Build history of the part. All positions in model axes, mm. Face numbers are marked on the shaded views. A direction names the side the tool comes from. Give positions to 0.01 mm unless a question says otherwise; leave off trailing zeros. Loops run counter-clockwise (first coordinate to the right, second up) from the corner with the lowest first, then second, coordinate; pieces in that order, holes last. Notation, with made-up numbers: (11.5, 9) -> (34.5, 9) arc R32 ccw to (34.5, 40) -> close; hole circle Ø11 at (58, -19.5). An arc over 180 degrees is marked (long way). One line per question, with ' | ' between items. Start each with the question number.
(1) Slice it at D-D, the plane z = 8. Write the cut outline in (x, y), then the cut area to 3 significant figures.
(2) Mould opens along X. For the marked faces 1, 2 and 3 say: pulls with the +X half, pulls with the -X half, needs draft (parallel to the pull), parting line crosses it, or undercut.
(3) Slice it at B-B, the plane z = 18. Write the cut outline in (x, y).
(4) 3-axis set-ups, long thin cutter, end or side, ignore diameter. For the marked faces 4 and 5: which of +Z, -Z, +X, -X, +Y, -Y reach the whole face in a straight line?
(5) Slice it at C-C, the plane x = 30. Write the cut outline in (y, z).
(6) Flat gauge pins, fed straight in: pin 1 Ø10 at (x, z) = (32.5, 14.5) entering from +Y; pin 2 Ø1.6 at (x, y) = (30, 1) entering from -Z; pin 3 Ø4 at (x, y) = (26.5, 20.5) entering from -Z; pin 4 Ø1 at (x, y) = (14.5, 12.5) entering from +Z. Where does each tip first touch, or does it go through?
(7) Slice it at A-A, the plane y = 23. Write the cut outline in (x, z).
(8) Drill centre lines: L1, parallel to X at y = 15, z = 16; L2, parallel to Z at x = 59.15, y = 56; L3, parallel to Z at x = 26.5, y = 25. Where is each one in solid material? Low to high. Write a range as from..to.
```python
from build123d import *

# Parameters (mm, degrees)
F0_W     = 60
F0_H     = 60
F1_DEPTH = 2
F3_DEPTH = 20
F5_DEPTH = 10
F6_R     = 2
F7_DEPTH = 69.4


with BuildPart() as f1:
    # F0 (on Top) → F1 (new body)
    with BuildSketch(Plane.XY):
        with Locations((30, 30)):
            Rectangle(F0_W, F0_H)
    extrude(amount=F1_DEPTH)

    # F2 (on face) → F3 (join)
    with BuildSketch(Plane.XY.offset(2)):
        Polygon((58, 2), (2, 2), (2, 60), (0, 60), (0, 0), (60, 0), (60, 60), (58, 60), align=None)
    extrude(amount=F3_DEPTH)

    # F4 (on face) → F5 (cut)
    with BuildSketch(Plane(origin=(0, 0, 0), x_dir=(1, 0, 0), z_dir=(0, 0, -1))):
        with BuildLine():
            Line((33, 2.964752), (27, 2.964752))
            Line((27, 2.964752), (27, -30))
            ThreePointArc((27, -30), (30, -33), (33, -30))
            Line((33, -30), (33, 2.964752))
        make_face()
    extrude(amount=-F5_DEPTH, mode=Mode.SUBTRACT)

    # F6 (on face) → F7 (cut)
    with BuildSketch(Plane(origin=(0, 0, 0), x_dir=(0, -1, 0), z_dir=(-1, 0, 0))):
        with Locations((-56, 18)):
            Circle(F6_R)
    extrude(amount=-F7_DEPTH, mode=Mode.SUBTRACT)


solid = f1.part
```
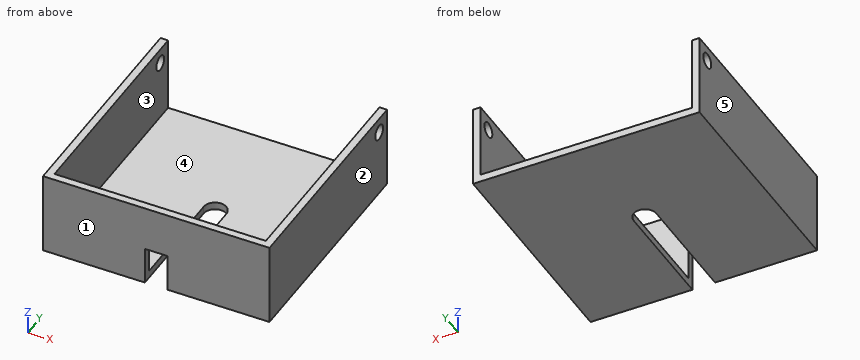
Final values:
1) outline: (0, 0) -> (27, 0) -> (27, 2) -> (2, 2) -> (2, 60) -> (0, 60) -> close; (33, 0) -> (60, 0) -> (60, 60) -> (58, 60) -> (58, 2) -> (33, 2) -> close | area: 340 mm2
2) face 1: needs draft | face 2: pulls with the +X half | face 3: undercut
3) outline: (0, 0) -> (60, 0) -> (60, 54) -> (58, 54) -> (58, 2) -> (2, 2) -> (2, 54) -> (0, 54) -> close; (0, 58) -> (2, 58) -> (2, 60) -> (0, 60) -> close; (58, 58) -> (60, 58) -> (60, 60) -> (58, 60) -> close
4) face 4: +Z, +Y | face 5: +Z, -Z, -X, +Y, -Y
5) outline: (0, 10) -> (2, 10) -> (2, 22) -> (0, 22) -> close; (33, 0) -> (60, 0) -> (60, 2) -> (33, 2) -> close
6) pin 1: y = 2 | pin 2: z = 10 | pin 3: z = 0 | pin 4: z = 2
7) outline: (0, 0) -> (27, 0) -> (27, 2) -> (2, 2) -> (2, 22) -> (0, 22) -> close; (33, 0) -> (60, 0) -> (60, 22) -> (58, 22) -> (58, 2) -> (33, 2) -> close
8) L1: 0..2, 58..60 | L2: 0..16, 20..22 | L3: 0..2
